from build123d import *

# Parameters (mm, degrees)
F1_DEPTH = 40.2336
F0_R     = 10.16
F2_DEPTH = 15.7734
F3_R     = 3.302


with BuildPart() as f1:
    # F0 (on Top) → F1 (new body)
    with BuildSketch(Plane.XY):
        with BuildLine():
            ThreePointArc((5.211817, -28.095686), (21.971098, -18.270235), (28.575, 0))
            ThreePointArc((28.575, 0), (21.971098, 18.270235), (5.211817, 28.095686))
            ThreePointArc((5.211817, 28.095686), (-28.575, 0), (5.211817, -28.095686))
        make_face()
        with BuildLine():
            ThreePointArc((-13.447765, 4.826), (0, 14.2875), (13.447765, 4.826))
            Line((13.447765, 4.826), (18.5293, 4.826))
            Line((18.5293, 4.826), (18.5293, -4.826))
            Line((18.5293, -4.826), (13.447765, -4.826))
            ThreePointArc((13.447765, -4.826), (0, -14.2875), (-13.447765, -4.826))
            Line((-13.447765, -4.826), (-18.5293, -4.826))
            Line((-18.5293, -4.826), (-18.5293, 4.826))
            Line((-18.5293, 4.826), (-13.447765, 4.826))
        make_face(mode=Mode.SUBTRACT)
        with BuildLine():
            ThreePointArc((-13.447765, -4.826), (-14.2875, 0), (-13.447765, 4.826))
            Line((-13.447765, 4.826), (-18.5293, 4.826))
            Line((-18.5293, 4.826), (-18.5293, -4.826))
            Line((-18.5293, -4.826), (-13.447765, -4.826))
        make_face()
    extrude(amount=F1_DEPTH)

    # F0 (on Top) → F2 (join)
    with BuildSketch(Plane.XY):
        with BuildLine():
            ThreePointArc((5.211817, 28.095686), (21.971098, 18.270235), (28.575, 0))
            ThreePointArc((28.575, 0), (21.971098, -18.270235), (5.211817, -28.095686))
            Line((5.211817, -28.095686), (53.975, -19.05))
            ThreePointArc((53.975, -19.05), (67.445384, -13.470384), (73.025, 0))
            ThreePointArc((73.025, 0), (67.445384, 13.470384), (53.975, 19.05))
            Line((53.975, 19.05), (5.211817, 28.095686))
        make_face()
        with Locations((53.975, 0)):
            Circle(F0_R, mode=Mode.SUBTRACT)
    extrude(amount=F2_DEPTH)

    # F3
    f3_edges = [f1.edges().sort_by_distance(p)[0] for p in [
        (-5.211817, 28.095686, 40.2336),
    ]]
    fillet(f3_edges, radius=F3_R)


solid = f1.part
Work out the finished part from the listing and answer in its coordinate system (mm). A direction names the side the tool comes from. Round coordinates to 2 decimals unless told otherwise and drop trailing zeros. Order: outer loops, then holes, each group sorted by start corner. A loop starts at its lowest first (then second) coordinate and runs counter-clockwise, first axis right, second up. Notation, with made-up numbers: M -18.5,85 L -0.5,85 A11 cw -0.5,96 Z; hole C 88.25,10 d2. An arc over 180 degrees is marked long. Put each result on its own line as item: value. Start each with the question number.
Q1. Section C-C, the plane y = -7 is taken. Give the number of separate pieces and of enclosed holes in the cut face, and give its area (3 significant figures).
Q2. A tool of negligible diameter and unlimited length cuts with its end or side. For faces 1 (the flat face through (18.529, 0, 20)), 2 (the flat face through (22, 0, 0)), from which of +Z, -Z, +X, -X, +Y, -Y can it reach the whole face along a straight path? Write none if from no direction.
Q3. Section B-B, the plane x = 55.5 is taken. Write down the section's boundary in (y, z).
Q4. Flat-ended cylindrical pins translate along their axes: pin 1 (2.5 mm diameter, centred on x = 15, z = 12, fed in from +Y); pin 2 (8 mm diameter, centred on x = 14.5, z = 20, fed in from -Y); pin 3 (3 mm diameter, centred on x = 13.5, z = 30, fed in from -Y). Find the tip coordinate at first contact, or state that the pin passes through.
Q5. For a pull along Y with two mould halves and no side action, classify faces 3 (the flat face through (39, 0, 15.773)), 4 (the flat face through (29.252, -23.636, 7.776)), 5 (the flat face through (29.93, 23.51, 7.78)), 6 (the flat face through (16, 4.826, 20)) as pulls with the +Y half, pulls with the -Y half, needs draft (parallel to the pull), parting line crosses it, or undercut.
Q6. Section D-D, the plane x = 35 is taken. Write down the section's boundary in (y, z), and give its area (3 significant figures).
Q7. Straight lines are drawn through the part: L1, parallel to X at y = 9, z = 4.5; L2, parallel to Y at x = 4, z = 30; L3, parallel to Y at x = 45, z = 9. For each, find the intervals that lie inside material, in ascending order. Write a range as [from, to].
Findings below:
1. separate pieces: 3
1. enclosed holes: 0
1. area: 1,680 mm^2
2. face 1: +Z, -Z
2. face 2: -Z, +X, -X, +Y, -Y
3. outline: M -18.99,0 L -10.04,0 L -10.04,15.77 L -18.99,15.77 Z; M 10.04,0 L 18.99,0 L 18.99,15.77 L 10.04,15.77 Z
4. pin 1: stops at y = 26.51
4. pin 2: stops at y = -26.58
4. pin 3: stops at y = -25.93
5. face 3: needs draft
5. face 4: pulls with the -Y half
5. face 5: pulls with the +Y half
5. face 6: undercut
6. outline: M -22.57,0 L 22.57,0 L 22.57,15.77 L -22.57,15.77 Z
6. area: 712 mm^2
7. L1: x = [-27.12, -11.1], [11.1, 49.26], [58.69, 70.76]
7. L2: y = [-28.29, -13.72], [13.72, 28.29]
7. L3: y = [-20.71, -4.76], [4.76, 20.71]
